Verification items for this drawing (mm, ordinates from the low corner). Give positions to 0.01 mm unless a question says otherwise; leave off trailing zeros. Write each loop counter-clockwise with the first axis right and the second up, starting at its lowest first coordinate (ties: lowest second). Pieces come first, ordered by that corner, then holes. Notation, with made-up numbers: (10, 36) -> (69, 36) arc R20 ccw to (69, 60) -> close; hole circle Ø3 at (86.5, 42). An arc over 180 degrees is marked (long way). Write item = value, one per line.
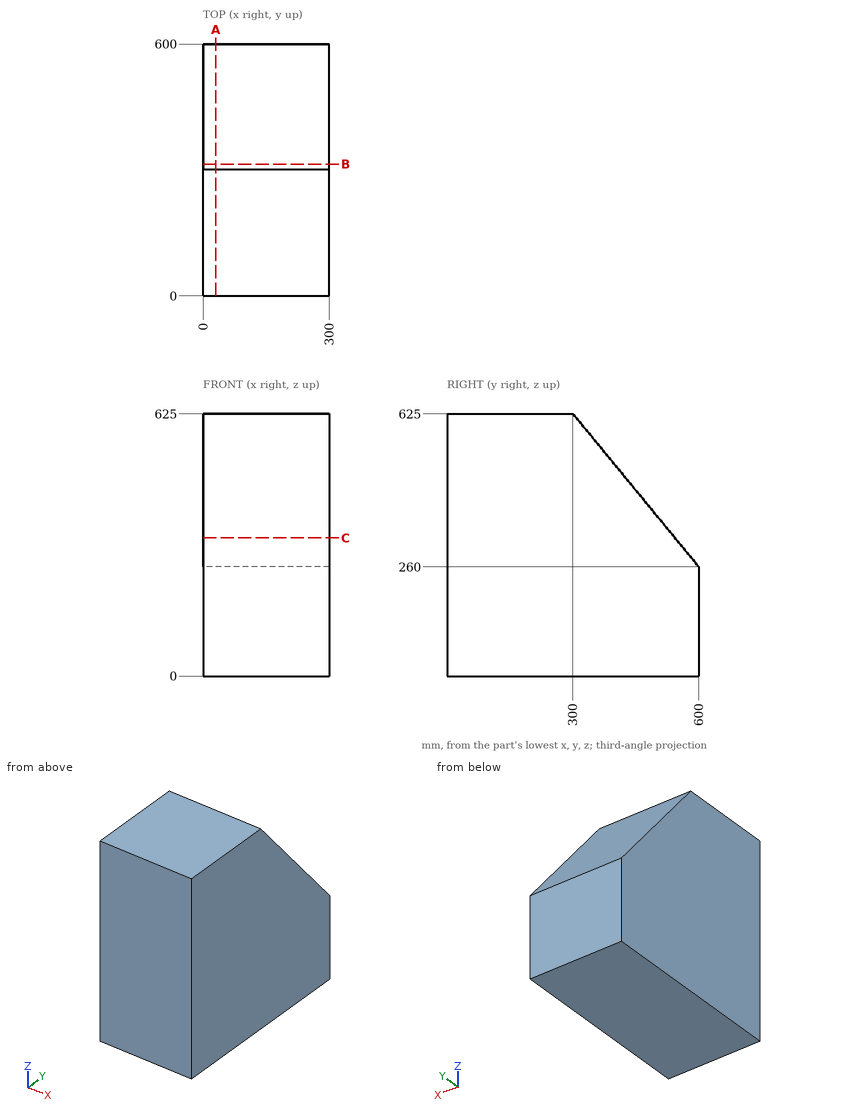
Item 1: Sectioned sample at A-A on x = 30.5. Record the cut outline in (y, z), then the cut area to 3 significant figures.
Response values:
outline = (0, 0) -> (600, 0) -> (600, 260) -> (300, 625) -> (0, 625) -> close
area = 320,000 mm^2
Item 2: Material ranges on line 1 (Z direction, x = 133, y = 528); line 2 (Y direction, x = 272.5, z = 398); line 3 (Y direction, x = 145.5, z = 459), recorded low to high.
Response values:
line_1 = 0 to 347.6
line_2 = 0 to 486.58
line_3 = 0 to 436.44
Item 3: Sectioned sample at C-C on z = 329. Record the cut outline in (x, y).
Response values:
outline = (0, 0) -> (300, 0) -> (300, 543.29) -> (0, 543.29) -> close
Item 4: Sectioned sample at B-B on y = 314. Record the cut outline in (x, z).
Response values:
outline = (0, 0) -> (300, 0) -> (300, 607.97) -> (0, 607.97) -> close
